```python
from build123d import *

# Parameters (mm, degrees)
SKETCH1_W           = 29
SKETCH1_H           = 25
BOSS_EXTRUDE1_DEPTH = 37
SKETCH2_W           = 27
SKETCH2_H           = 35
CUT_EXTRUDE1_DEPTH  = 37
FILLET1_R           = 2
SKETCH3_R           = 1.5
SKETCH3_R_2         = 4
CUT_EXTRUDE2_DEPTH  = 52.874849397
FILLET3_R           = 12
FILLET4_R           = 12
SKETCH5_R           = 1.5
SKETCH5_R_2         = 4
CUT_EXTRUDE3_DEPTH  = 53.182372503


with BuildPart() as part:
    # Sketch1 → Boss-Extrude1 (new body)
    with BuildSketch(Plane(origin=(0, 0, 0), x_dir=(1, 0, 0), z_dir=(0, 1, 0))):
        with Locations((14.5, 12.5)):
            Rectangle(SKETCH1_W, SKETCH1_H)
    extrude(amount=BOSS_EXTRUDE1_DEPTH)

    # Sketch2 → Cut-Extrude1 (cut)
    with BuildSketch(Plane.XY):
        with Locations((15.5, 19.5)):
            Rectangle(SKETCH2_W, SKETCH2_H)
    extrude(amount=-CUT_EXTRUDE1_DEPTH, mode=Mode.SUBTRACT)

    # Fillet1
    fillet1_edges = [part.edges().sort_by_distance(p)[0] for p in [
        (0, 0, -12.5),
    ]]
    fillet(fillet1_edges, radius=FILLET1_R)

    # Sketch3 → Cut-Extrude2 (cut, through all)
    with BuildSketch(Plane(origin=(0, 2, 0), x_dir=(1, 0, 0), z_dir=(0, 1, 0))):
        with Locations(Location((23.5, 12.5, 0), (0, 0, 180))):
            Circle(SKETCH3_R)
        with Locations(Location((17, 12.5, 0), (0, 0, 180))):
            Circle(SKETCH3_R_2)
        with Locations(Location((10.5, 12.5, 0), (0, 0, 180))):
            Circle(SKETCH3_R)
        with Locations(Location((17, 19, 0), (0, 0, 180))):
            Circle(SKETCH3_R)
        with Locations((17, 6)):
            Circle(SKETCH3_R)
    extrude(amount=-CUT_EXTRUDE2_DEPTH, mode=Mode.SUBTRACT)

    # Fillet3
    fillet3_edges = [part.edges().sort_by_distance(p)[0] for p in [
        (29, 1, -25),
        (29, 1, 0),
    ]]
    fillet(fillet3_edges, radius=FILLET3_R)

    # Fillet4
    fillet4_edges = [part.edges().sort_by_distance(p)[0] for p in [
        (1, 37, -25),
        (1, 37, 0),
    ]]
    fillet(fillet4_edges, radius=FILLET4_R)

    # Sketch5 → Cut-Extrude3 (cut, through all)
    with BuildSketch(Plane(origin=(2, 0, 0), x_dir=(0, 0, -1), z_dir=(1, 0, 0))):
        with Locations(Location((12.5, 31.5, 0), (0, 0, 90))):
            Circle(SKETCH5_R)
        with Locations(Location((12.5, 25, 0), (0, 0, 90))):
            Circle(SKETCH5_R_2)
        with Locations(Location((6, 25, 0), (0, 0, 90))):
            Circle(SKETCH5_R)
        with Locations(Location((19, 25, 0), (0, 0, 270))):
            Circle(SKETCH5_R)
        with Locations(Location((12.5, 18.5, 0), (0, 0, 90))):
            Circle(SKETCH5_R)
    extrude(amount=-CUT_EXTRUDE3_DEPTH, mode=Mode.SUBTRACT)


solid = part.part
```
Can you work these out from the model? Positions are in its coordinate system, mm. A direction names the side the tool comes from. Round coordinates to 2 decimals unless told otherwise and drop trailing zeros. Order: outer loops, then holes, each group sorted by start corner. A loop starts at its lowest first (then second) coordinate and runs counter-clockwise, first axis right, second up.
(1) If we section it at B-B (z = -12.5): Count the separate pieces of the cut face and the enclosed holes in it, plus the area to 3 significant figures.
Results are:
separate pieces: 7
enclosed holes: 0
area: 71.1 mm2
(2) We'd pull the mould along X, two halves only. Please class faces 3 (the face through (0, 15, -12)), 4 (the face through (1, 21.8, -14.9)), 5 (the face through (15.5, 1.01, -6.07)): +X half, -X half, draft (parallel to the pull), parting line (faces both ways), or undercut.
Results are:
face 3: -X half
face 4: draft
face 5: undercut
(3) If I drill on L1, parallel to Z at x = 1.35, y = 25; L2, parallel to Z at x = 1.4, y = 18.5; L3, parallel to X at y = 22, z = -1.25, over which ranges is the centre line in solid material (lowest first)?
Results are:
L1: z = -25 to -20.5, -17.5 to -16.5, -8.5 to -7.5, -4.5 to 0
L2: z = -25 to -14, -11 to 0
L3: x = 0 to 2
(4) I'm going to push flat-ended pins straight in: pin 1 (2.5 mm diameter, centred on x = 17, z = -6, fed in from -Y); pin 2 (1 mm diameter, centred on y = 28.5, z = -18.5, fed in from -X); pin 3 (5 mm diameter, centred on y = 24, z = -8.5, fed in from +X). Where does each tip first touch, or does it pass through?
Results are:
pin 1: passes through
pin 2: stops at x = 0
pin 3: stops at x = 2
(5) On a 3-axis mill with a long thin cutter (end or side, diameter ignored), from which of +Z, -Z, +X, -X, +Y, -Y can I reach the whole of each face in a straight line? I mean faces 1 (the face through (1.5, 7.8, -25)), 2 (the face through (12.3, 2, -12.3)). Say none if no direction works.
Results are:
face 1: -Z, +X, -X, +Y, -Y
face 2: +Z, -Z, +X, +Y
(6) If we section it at A-A (x = 10.5): Please give me the cut outline in (y, z).
Results are:
outline: (0, -25) - (2, -25) - (2, -14) - (0, -14) - close; (0, -11) - (2, -11) - (2, 0) - (0, 0) - close
(7) If we section it at D-D (z = -15.25): Please give me the cut outline in (x, y), plus the area to 3 significant figures.
Results are:
outline: (0, 2) arc R2 ccw to (2, 0) - (14.1, 0) - (14.1, 2) - (2, 2) - (2, 22.1) - (0, 22.1) - close; (0, 27.9) - (2, 27.9) - (2, 36.79) - (0, 36.79) - close; (19.9, 0) - (28.79, 0) - (28.79, 2) - (19.9, 2) - close
area: 103 mm2
